```python
from build123d import *

# Parameters (mm, degrees)
F1_DEPTH = 6
F2_R     = 2.883162
F3_DEPTH = 30


with BuildPart() as f1:
    # F0 (on Front) → F1 (new body)
    with BuildSketch(Plane.XZ):
        with BuildLine():
            Line((-28.426227, 0), (-6, 0))
            ThreePointArc((-6, 0), (-1.757359, 1.757359), (0, 6))
            Line((0, 6), (0, 29.860658))
            ThreePointArc((0, 29.860658), (-1.757359, 34.103298), (-6, 35.860658))
            Line((-6, 35.860658), (-28.426227, 35.860658))
            ThreePointArc((-28.426227, 35.860658), (-32.668868, 34.103298), (-34.426227, 29.860658))
            Line((-34.426227, 29.860658), (-34.426227, 6))
            ThreePointArc((-34.426227, 6), (-32.668868, 1.757359), (-28.426227, 0))
        make_face()
    extrude(amount=F1_DEPTH)

    # F2 (on face) → F3 (cut)
    with BuildSketch(Plane.XZ.offset(6)):
        with Locations((-16.926229, 17.069673)):
            Circle(F2_R)
    extrude(amount=-F3_DEPTH, mode=Mode.SUBTRACT)


solid = f1.part
```
Input: part model. Units: mm. Frame: model coordinates. Give positions to 0.01 mm unless a question says otherwise; leave off trailing zeros. Order: outer loops, then holes, each group sorted by start corner. A loop starts at its lowest first (then second) coordinate and runs counter-clockwise, first axis right, second up. Notation, with made-up numbers: (76, 76) - (108, 76) arc R31 ccw to (108, 115) - close; hole circle Ø2 at (-12, 47). An arc over 180 degrees is marked (long way). Put each result on its own line as item: value.
Item 1: Ray query, L1, parallel to Z at x = -17, y = -3.6; L2, parallel to X at y = -3.6, z = 18; L3, parallel to Z at x = -28.5, y = -0.65. Return the intervals inside material, ascending. Write a range as from..to.
Found:
L1: z = 0..14.19, 19.95..35.86
L2: x = -34.43..-19.66, -14.2..0
L3: z = 0..35.86
Item 2: Draft query along Z for faces 1 (the flat face through (-17, -3, 0)), 2 (the flat face through (-17, -3, 35.861)), 3 (the cylindrical face through (-19.2, -3, 15.3)). Return one class per face: +Z half, -Z half, draft (parallel to the pull), parting line (faces both ways), or undercut.
Found:
face 1: -Z half
face 2: +Z half
face 3: undercut
Item 3: Section query C-C, the plane x = -2. Return loops of the section in (y, z), then the cut area to 3 significant figures.
Found:
outline: (-6, 1.53) - (0, 1.53) - (0, 34.33) - (-6, 34.33) - close
area: 197 mm^2
Item 4: Section query A-A, the plane x = -17. Return loops of the section in (y, z), then the cut area to 3 significant figures.
Found:
outline: (-6, 0) - (0, 0) - (0, 14.19) - (-6, 14.19) - close; (-6, 19.95) - (0, 19.95) - (0, 35.86) - (-6, 35.86) - close
area: 181 mm^2
Item 5: Section query B-B, the plane y = -2.5. Return loops of the section in (x, z).
Found:
outline: (-34.43, 6) arc R6 ccw to (-28.43, 0) - (-6, 0) arc R6 ccw to (0, 6) - (0, 29.86) arc R6 ccw to (-6, 35.86) - (-28.43, 35.86) arc R6 ccw to (-34.43, 29.86) - close; hole circle Ø5.77 at (-16.93, 17.07)
Item 6: Section query D-D, the plane z = 32. Return loops of the section in (x, y).
Found:
outline: (-34.03, -6) - (-0.39, -6) - (-0.39, 0) - (-34.03, 0) - close
